For this review, take the finished solid that the model builds, in its own axes (mm). Face numbers are marked on the shaded views. Coordinates: 2 decimals unless noted, no trailing zeros. Loops run counter-clockwise (first coordinate to the right, second up) from the corner with the lowest first, then second, coordinate; pieces in that order, holes last. Notation, with made-up numbers: M -38,66.25 L -1,66.25 A13 cw -1,79.25 Z; hole C -31.5,6.25 d4. An arc over 180 degrees is marked long. Answer as a JSON object with one key per item and string values. Group by question number.
Item 1: Insertion check: pin 1 (4 mm diameter, centred on x = 26.63, y = 12.1, fed in from -Z); pin 2 (6 mm diameter, centred on y = -3, z = -13, fed in from +X). Each pin has a flat end and moves straight along its axis. Give the tip position at first contact, or say it passes through.
Item 2: Add section B-B (z = -3). State the section outline as (x, y) points, then the cut area to 3 significant figures.
Item 3: Mouldability with a two-part tool opening along X and no side actions: class the marked faces 1, 2, 3 and 4 as +X half, -X half, draft (parallel to the pull), parting line (faces both ways), or undercut.
Item 4: Add section D-D (y = -7.5). State the section outline as (x, z) points, then the cut area to 3 significant figures.
Item 5: Add section C-C (x = 0). State the section outline as (y, z) points.
Item 6: Wall thickness on L1, parallel to X at y = 11.25, z = -3.75; L2, parallel to Y at x = 0, z = -6.75; L3, parallel to Z at x = -20, y = 2.75: over which ranges is each line inside the solid? List them lowest first. Write a range as from..to.
Item 7: Add section A-A (y = 0). State the section outline as (x, z) points.
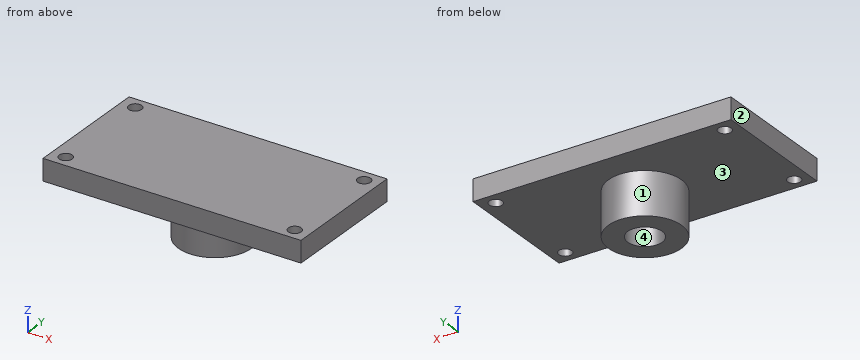
from build123d import *

# Parameters (mm, degrees)
F2_W     = 60
F2_H     = 30
F2_R     = 1.5
F3_DEPTH = 5
F1_R     = 8.5
F1_R_2   = 4
F4_DEPTH = 15


with BuildPart() as f3:
    # F2 (on face) → F3 (new body)
    with BuildSketch(Plane.XY):
        Rectangle(F2_W, F2_H)
        with Locations((-26.629558, -12.103098)):
            Circle(F2_R, mode=Mode.SUBTRACT)
        with Locations((26.629558, -12.103098)):
            Circle(F2_R, mode=Mode.SUBTRACT)
        with Locations((-26.629558, 12.103098)):
            Circle(F2_R, mode=Mode.SUBTRACT)
        with Locations((26.629558, 12.103098)):
            Circle(F2_R, mode=Mode.SUBTRACT)
    extrude(amount=-F3_DEPTH)

    # F1 (on face) → F4 (join)
    with BuildSketch(Plane.XY):
        Circle(F1_R)
        Circle(F1_R_2, mode=Mode.SUBTRACT)
    extrude(amount=-F4_DEPTH)


solid = f3.part
From the geometry:
{
 "1": {"pin 1": "stops at z = -5", "pin 2": "stops at x = 8.5"},
 "2": {"outline": "M -30,-15 L 30,-15 L 30,15 L -30,15 Z; hole C -26.63,-12.1 d3; hole C -26.63,12.1 d3; hole C 26.63,-12.1 d3; hole C 26.63,12.1 d3", "area": "1,770 mm²"},
 "3": {"face 1": "parting line", "face 2": "-X half", "face 3": "draft", "face 4": "undercut"},
 "4": {"outline": "M -30,-5 L -4,-5 L -4,-15 L 4,-15 L 4,-5 L 30,-5 L 30,0 L -30,0 Z", "area": "380 mm²"},
 "5": {"outline": "M -15,-5 L -8.5,-5 L -8.5,-15 L -4,-15 L -4,-5 L 4,-5 L 4,-15 L 8.5,-15 L 8.5,-5 L 15,-5 L 15,0 L -15,0 Z"},
 "6": {"L1": "x = -30..-27.86, -25.4..25.4, 27.86..30", "L2": "y = -8.5..-4, 4..8.5", "L3": "z = -5..0"},
 "7": {"outline": "M -30,-5 L -8.5,-5 L -8.5,-15 L -4,-15 L -4,-5 L 4,-5 L 4,-15 L 8.5,-15 L 8.5,-5 L 30,-5 L 30,0 L -30,0 Z"}
}
